Model file for the job. Use its own axes, mm. Coordinates: 2 decimals unless noted, no trailing zeros. Write each loop counter-clockwise with the first axis right and the second up, starting at its lowest first coordinate (ties: lowest second). Pieces come first, ordered by that corner, then holes. Notation, with made-up numbers: (12.25, 51) -> (30.25, 51) arc R12 ccw to (30.25, 57) -> close; hole circle Ø6 at (0.5, -21.75). An arc over 180 degrees is marked (long way). Answer as a JSON object with one key per item and string values. Group by question number.
from build123d import *

# Parameters (mm, degrees)
SKETCH_1_R          = 7.5
EXTRUDE_1_DEPTH     = 7
SKETCH_2_R          = 5.25
CUT_EXTRUDE_1_DEPTH = 6
SKETCH_3_R          = 6.5
CUT_EXTRUDE_2_DEPTH = 5
FILLET_1_R          = 0.5


with BuildPart() as part:
    # 草图1 → 凸台-拉伸1 (new body)
    with BuildSketch(Plane.XY):
        Circle(SKETCH_1_R)
    extrude(amount=EXTRUDE_1_DEPTH)

    # 草图2 → 切除-拉伸1 (cut)
    with BuildSketch(Plane.XY.offset(7)):
        Circle(SKETCH_2_R)
    extrude(amount=-CUT_EXTRUDE_1_DEPTH, mode=Mode.SUBTRACT)

    # 草图3 → 切除-拉伸2 (cut)
    with BuildSketch(Plane.XY.offset(1)):
        Circle(SKETCH_3_R)
    extrude(amount=CUT_EXTRUDE_2_DEPTH, mode=Mode.SUBTRACT)

    # 圆角1
    fillet_1_edges = [part.edges().sort_by_distance(p)[0] for p in [
        (-7.5, 0, 0),
        (-7.5, 0, 7),
        (-5.25, 0, 7),
    ]]
    fillet(fillet_1_edges, radius=FILLET_1_R)


solid = part.part
(1) Cut at A-A on x = 0. List the corners of the cut face in (y, z), plus the area to 3 significant figures.
(2) Pull direction Z, two halves, no side cores. Call faces 1 (the face through (0, 0, 1)), 2 (the face through (-5.158, -3.955, 3.465)), 3 (the face through (5, 1.6, 6.3)), 4 (the face through (-1, 6, 7)): released by +Z, released by -Z, zero draft, split by the parting line, or undercut.
(3) Wall check: probe 1 along Y at (x, z) = (0, 6.3); probe 2 along Y at (x, z) = (0, 3.7); probe 3 along Z at (x, y) = (1.75, -6). Give the ranges that are in metal, low to high.
(4) Cut at C-C on z = 2.5. List the corners of the cut face in (x, y).
(5) Cut at D-D on z = 0.75. List the corners of the cut face in (x, y).
(6) Pin check, flat tips, straight feed: pin 1 (6 mm diameter, centred on x = 0, y = -3.5, fed in from -Z); pin 2 (1 mm diameter, centred on y = 4, z = 3.5, fed in from +X); pin 3 (3 mm diameter, centred on x = 4, z = 5, fed in from -Y). Stop position of each tip, or through.
Results found:
{
 "1": {"outline": "(-7.5, 0.5) arc R0.5 ccw to (-7, 0) -> (7, 0) arc R0.5 ccw to (7.5, 0.5) -> (7.5, 6.5) arc R0.5 ccw to (7, 7) -> (5.75, 7) arc R0.5 ccw to (5.25, 6.5) -> (5.25, 6) -> (6.5, 6) -> (6.5, 1) -> (-6.5, 1) -> (-6.5, 6) -> (-5.25, 6) -> (-5.25, 6.5) arc R0.5 ccw to (-5.75, 7) -> (-7, 7) arc R0.5 ccw to (-7.5, 6.5) -> close", "area": "29.2 mm²"},
 "2": {"face 1": "undercut", "face 2": "undercut", "face 3": "zero draft", "face 4": "released by +Z"},
 "3": {"probe 1": "y = -7.5 to -5.25, 5.25 to 7.5", "probe 2": "y = -7.5 to -6.5, 6.5 to 7.5", "probe 3": "z = 0 to 1, 6 to 7"},
 "4": {"outline": "circle Ø15 at (0, 0); hole circle Ø13 at (0, 0)"},
 "5": {"outline": "circle Ø15 at (0, 0)"},
 "6": {"pin 1": "stops at z = 0", "pin 2": "stops at x = 6.63", "pin 3": "stops at y = -7.07"}
}
